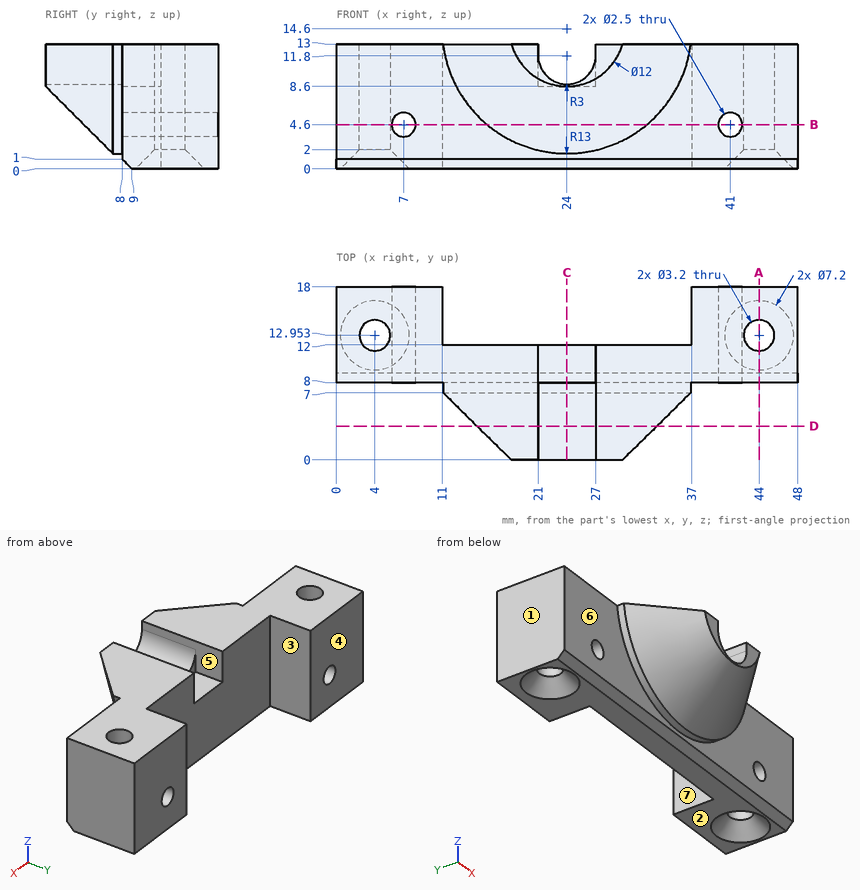
Could you check a few things on this drawing? It's one solid part, dimensions in mm from its lowest x, y, z. A direction names the side the tool comes from. Round coordinates to 2 decimals unless told otherwise and drop trailing zeros. Write each loop counter-clockwise with the first axis right and the second up, starting at its lowest first coordinate (ties: lowest second). Pieces come first, ordered by that corner, then holes. Notation, with made-up numbers: (-5, 88) -> (19, 88) arc R18 ccw to (19, 123) -> close; hole circle Ø11 at (-23, -23). An arc over 180 degrees is marked (long way). Use a Markdown table: item, result.
1. We'd pull the mould along X, two halves only. Please class the marked faces 1, 2 and 3: +X half, -X half, draft (parallel to the pull), parting line (faces both ways), or undercut.
Answer key:
| item | result |
|---|---|
| face 1 | -X half |
| face 2 | draft |
| face 3 | undercut |
2. Which directions (+Z, -Z, +X, -X, +Y, -Y) give clear straight access to the entire face, cutting with the end or side of a thin tool? Please do the marked faces 4, 5, 6 and 7.
Answer key:
| item | result |
|---|---|
| face 4 | +Z, -Z, +X, -X, +Y |
| face 5 | +Z, +Y |
| face 6 | -Z, -Y |
| face 7 | +Z, -Z, +Y |
3. If we section it at C-C (x = 24): List the corners of the cut face in (y, z) for me.
Answer key:
| item | result |
|---|---|
| outline | (0, 8.6) -> (7, 1.6) -> (8, 1.6) -> (8, 1) -> (9, 0) -> (12, 0) -> (12, 8.6) -> (8, 8.6) -> (8, 8.8) -> (0, 8.8) -> close |
4. If we section it at A-A (x = 44): List the corners of the cut face in (y, z) for me, then the cut area to 3 significant figures.
Answer key:
| item | result |
|---|---|
| outline | (8, 1) -> (9, 0) -> (9.35, 0) -> (11.35, 2) -> (11.35, 13) -> (8, 13) -> close; (14.55, 2) -> (16.55, 0) -> (18, 0) -> (18, 13) -> (14.55, 13) -> close |
| area | 83.9 mm^2 |
5. For pin 1 Ø1.2 at (x, y) = (24.5, 10.5) entering from +Z; pin 2 Ø3.5 at (x, z) = (27, 5) entering from -Y; pin 3 Ø3.5 at (y, z) = (4, 11.5) entering from +X; pin 4 Ø1 at (x, z) = (6.5, 5) entering from +Y, each with a flat end and sliding along its axis, tell me the tip position at first contact or that it passes through.
Answer key:
| item | result |
|---|---|
| pin 1 | stops at z = 8.6 |
| pin 2 | stops at y = 2.31 |
| pin 3 | stops at x = 35.39 |
| pin 4 | passes through |
6. If we section it at D-D (y = 3.5): List the corners of the cut face in (x, z) for me.
Answer key:
| item | result |
|---|---|
| outline | (14.64, 13) arc R9.5 ccw to (33.36, 13) -> (27, 13) -> (27, 11.8) arc R3 cw to (21, 11.8) -> (21, 13) -> close |
7. If we section it at B-B (z = 4.6): State how many separate pieces and enclosed holes the cut face has, then the cut area to 3 significant figures.
Answer key:
| item | result |
|---|---|
| separate pieces | 3 |
| enclosed holes | 2 |
| area | 307 mm^2 |
8. Please list where these lines run through material, in increasing order: probe 1 along Y at (x, z) = (44, 8); probe 2 along X at (y, z) = (8.5, 5.5); probe 3 along X at (y, z) = (8.5, 9.5).
Answer key:
| item | result |
|---|---|
| probe 1 | y = 8 to 11.35, 14.55 to 18 |
| probe 2 | x = 0 to 6.13, 7.87 to 40.13, 41.87 to 48 |
| probe 3 | x = 0 to 21, 27 to 48 |
